The listing builds one solid part. Answer for the finished solid, in the listing's coordinates (mm). Round coordinates to 2 decimals unless told otherwise and drop trailing zeros. Write each loop counter-clockwise with the first axis right and the second up, starting at its lowest first coordinate (ties: lowest second). Pieces come first, ordered by that corner, then holes. Notation, with made-up numbers: (80.5, 46) -> (87.5, 46) arc R31 cw to (87.5, 85) -> close; hole circle Ø11 at (72.5, 66.5). An arc over 180 degrees is marked (long way). Write each question's results on one line, items separated by ' | '. Start each with the question number.
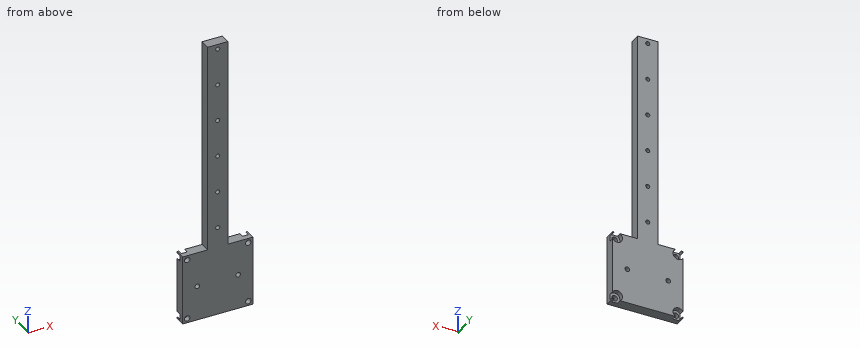
```python
from build123d import *

# Parameters (mm, degrees)
EXTRUDE1_DEPTH                 = 6.35
LPATTERN1_COUNT                = 6
LPATTERN1_PITCH                = 22.9
CBORE_FOR_M3_SHCS1_D           = 3.4
CBORE_FOR_M3_SHCS1_CBORE_D     = 6.5
CBORE_FOR_M3_SHCS1_CBORE_DEPTH = 3
LPATTERN2_COUNT                = 2
LPATTERN2_PITCH                = 37.5
LPATTERN2_COUNT_DIR2           = 2
LPATTERN2_PITCH_DIR2           = 37.5
F_2_9_2_9_DIAMETER_HOLE1_D     = 2.9


with BuildPart() as part:
    # Sketch2 → Extrude1 (new body)
    with BuildSketch(Plane(origin=(0, 0, 0), x_dir=(1, 0, 0), z_dir=(0, 1, 0))):
        Polygon((-6.25, -21.5), (-21.5, -21.5), (-21.5, 21.5), (21.5, 21.5), (21.5, -21.5), (6.25, -21.5), (6.25, -151.5), (-6.25, -151.5), align=None)
    extrude(amount=EXTRUDE1_DEPTH)

    # Sketch5 → M3x0.5 Tapped Hole1 (revolve, cut)
    with BuildSketch(Plane(origin=(0, 6.35, 148.5), x_dir=(0, 0, 1), z_dir=(1, 0, 0))):
        Polygon((0, 0), (0, 8.251075774), (1.25, 7.5), (1.25, 0), align=None)
    m3x0_5_tapped_hole1 = revolve(axis=Axis((0, 12.7, 148.5), (0, -1, 0)), mode=Mode.SUBTRACT)

    # LPattern1: M3x0.5 Tapped Hole1 ×6
    with Locations(*[(0, 0, -i * LPATTERN1_PITCH) for i in range(1, LPATTERN1_COUNT)]):
        add(m3x0_5_tapped_hole1, mode=Mode.SUBTRACT)

    # CBORE for M3 SHCS1 (through all)
    with Locations(Plane(origin=(-18.75, 6.35, -18.75), x_dir=(0, 0, 1), z_dir=(0, 1, 0))):
        with Locations((0, 0)):
            cbore_for_m3_shcs1 = CounterBoreHole(CBORE_FOR_M3_SHCS1_D / 2, CBORE_FOR_M3_SHCS1_CBORE_D / 2, CBORE_FOR_M3_SHCS1_CBORE_DEPTH)

    # LPattern2: CBORE for M3 SHCS1 2 × 2
    with Locations(*[(i * LPATTERN2_PITCH, 0, j * LPATTERN2_PITCH_DIR2) for i in range(LPATTERN2_COUNT) for j in range(LPATTERN2_COUNT_DIR2) if (i, j) != (0, 0)]):
        add(cbore_for_m3_shcs1, mode=Mode.SUBTRACT)

    # Ø2.9 (2.9) Diameter Hole1 (through all)
    with Locations(Plane(origin=(-12.5, 6.35, 0), x_dir=(0, 0, 1), z_dir=(0, 1, 0))):
        with Locations((0, 0), (0, 25)):
            Hole(F_2_9_2_9_DIAMETER_HOLE1_D / 2)


solid = part.part
```
Q1. Each of these flat-tipped pins is pushed along its axis until it touches: pin 1 (8 mm diameter, centred on x = -11.5, z = 112.5, fed in from +Y); pin 2 (1.8 mm diameter, centred on x = 18, z = -18, fed in from +Y); pin 3 (1 mm diameter, centred on y = 1.5, z = 68, fed in from +X); pin 4 (3 mm diameter, centred on x = -12, y = 3, fed in from +Z). Where does it stop, or does it pass through?
Q2. The part is cut by section D-D, the plane x = 18.75. Write down the section's boundary in (y, z), then the cut area to 3 significant figures.
Q3. The part is cut by section B-B, the plane x = 12.5. Write down the section's boundary in (y, z).
Q4. Find the intervals of material crossed by line 1 (X direction, y = 1.45, z = -18.75); line 2 (X direction, y = 3.5, z = 0); line 3 (X direction, y = 2, z = 120.5), in increasing order.
Q5. The part is cut by section A-A, the plane z = 18.75. Write down the section's boundary in (x, y).
Q6. The part is cut by section C-C, the plane y = 2. State how many separate pieces and enclosed holes the cut face has, then the cut area to 3 significant figures.
Answers follow:
1) pin 1: through | pin 2: y = 3.35 | pin 3: x = 6.25 | pin 4: z = 21.5
2) outline: (0, -21.5) -> (3.35, -21.5) -> (3.35, -20.45) -> (0, -20.45) -> close; (0, -17.05) -> (3.35, -17.05) -> (3.35, -15.5) -> (6.35, -15.5) -> (6.35, 15.5) -> (3.35, 15.5) -> (3.35, 17.05) -> (0, 17.05) -> close; (0, 20.45) -> (3.35, 20.45) -> (3.35, 21.5) -> (0, 21.5) -> close | area: 214 mm^2
3) outline: (0, -21.5) -> (6.35, -21.5) -> (6.35, -1.45) -> (0, -1.45) -> close; (0, 1.45) -> (6.35, 1.45) -> (6.35, 21.5) -> (0, 21.5) -> close
4) line 1: -21.5 to -20.45, -17.05 to 17.05, 20.45 to 21.5 | line 2: -21.5 to -13.95, -11.05 to 11.05, 13.95 to 21.5 | line 3: -6.25 to 6.25
5) outline: (-21.5, 0) -> (-20.45, 0) -> (-20.45, 3.35) -> (-21.5, 3.35) -> close; (-17.05, 0) -> (17.05, 0) -> (17.05, 3.35) -> (15.5, 3.35) -> (15.5, 6.35) -> (-15.5, 6.35) -> (-15.5, 3.35) -> (-17.05, 3.35) -> close; (20.45, 0) -> (21.5, 0) -> (21.5, 3.35) -> (20.45, 3.35) -> close
6) separate pieces: 1 | enclosed holes: 12 | area: 3,400 mm^2
